Could you check a few things on this model? Use its own coordinates, in mm. A direction names the side the tool comes from. Coordinates: 2 decimals unless noted, no trailing zeros. Write each loop counter-clockwise with the first axis right and the second up, starting at its lowest first coordinate (ties: lowest second). Pieces come first, ordered by that corner, then holes.
```python
from build123d import *

# Parameters (mm, degrees)
SCHIZZO1_W                   = 12
SCHIZZO1_H                   = 21
SCHIZZO1_W_2                 = 21
SCHIZZO1_W_3                 = 15.1
SCHIZZO1_H_2                 = 15.1
ESTRUSIONE_ESTRUSIONE1_DEPTH = 15
SCHIZZO2_R                   = 1.5
TAGLIO_ESTRUSIONE1_DEPTH     = 15
SCHIZZO3_R                   = 1.5
TAGLIO_ESTRUSIONE2_DEPTH     = 15


with BuildPart() as part:
    # Schizzo1 → Estrusione-Estrusione1 (new body)
    # profile 1 of 2: a face of its own
    with BuildSketch(Plane(origin=(0, 0, 0), x_dir=(0, 0, -1), z_dir=(1, 0, 0))):
        with Locations((-16.5, 0)):
            Rectangle(SCHIZZO1_W, SCHIZZO1_H)
    # profile 2 of 2: a face of its own
    with BuildSketch(Plane(origin=(0, 0, 0), x_dir=(0, 0, -1), z_dir=(1, 0, 0))):
        Rectangle(SCHIZZO1_W_2, SCHIZZO1_H)
        Rectangle(SCHIZZO1_W_3, SCHIZZO1_H_2, mode=Mode.SUBTRACT)
    extrude(amount=ESTRUSIONE_ESTRUSIONE1_DEPTH)

    # Schizzo2 → Taglio-Estrusione1 (cut)
    with BuildSketch(Plane(origin=(0, 10.5, 0), x_dir=(1, 0, 0), z_dir=(0, 1, 0))):
        with Locations(Location((7.5, -15.5, 0), (0, 0, 270))):
            Circle(SCHIZZO2_R)
    extrude(amount=-TAGLIO_ESTRUSIONE1_DEPTH, mode=Mode.SUBTRACT)

    # Schizzo3 → Taglio-Estrusione2 (cut)
    with BuildSketch(Plane.XZ.offset(10.5)):
        with Locations(Location((7.5, 19.5, 0), (0, 0, 270))):
            Circle(SCHIZZO3_R)
    extrude(amount=-TAGLIO_ESTRUSIONE2_DEPTH, mode=Mode.SUBTRACT)


solid = part.part
```
1. If we mould it in two halves opening along Z, with no side actions, what happens to faces 6 (the face through (7, -10.5, 6)), 7 (the face through (6.6, -3.1, 20.7)), 8 (the face through (7, 0, -10.5))? For each: pulls with the +Z half, pulls with the -Z half, needs draft (parallel to the pull), parting line crosses it, or undercut.
Verdict:
face 6: needs draft
face 7: undercut
face 8: pulls with the -Z half
2. For pin 1 (2.5 mm diameter, centred on x = 7.5, z = 15.5, fed in from +Y); pin 2 (1.5 mm diameter, centred on x = 7.5, z = 19, fed in from -Y), each with a flat end and sliding along its axis, tell me the tip position at first contact or that it passes through.
Verdict:
pin 1: stops at y = -4.5
pin 2: stops at y = 4.5
3. Please list where these lines run through material, in increasing order: line 1 along Z through (x, y) = (5.5, -6.25); line 2 along Y through (x, z) = (0.5, -3); line 3 along X through (y, z) = (-2.75, 19.5).
Verdict:
line 1: z = -10.5 to -7.55, 7.55 to 22.5
line 2: y = -10.5 to -7.55, 7.55 to 10.5
line 3: x = 0 to 6, 9 to 15
4. I want a section at D-D on x = 3.5. Please give me the cut outline in (y, z).
Verdict:
outline: (-10.5, -10.5) - (10.5, -10.5) - (10.5, 22.5) - (-10.5, 22.5) - close; hole (-7.55, -7.55) - (7.55, -7.55) - (7.55, 7.55) - (-7.55, 7.55) - close
5. I want a section at B-B on z = 7. Please give me the cut outline in (x, y).
Verdict:
outline: (0, -10.5) - (15, -10.5) - (15, -7.55) - (0, -7.55) - close; (0, 7.55) - (15, 7.55) - (15, 10.5) - (0, 10.5) - close
6. I want a section at A-A on y = -5.25. Please give me the cut outline in (x, z), plus the area to 3 significant figures.
Verdict:
outline: (0, -10.5) - (15, -10.5) - (15, -7.55) - (0, -7.55) - close; (0, 7.55) - (15, 7.55) - (15, 22.5) - (0, 22.5) - close; hole circle Ø3 at (7.5, 19.5)
area: 261 mm2
7. On a 3-axis mill with a long thin cutter (end or side, diameter ignored), from which of +Z, -Z, +X, -X, +Y, -Y can I reach the whole of each face in a straight line? I mean faces 1 (the face through (8, 4.5, 20)), 2 (the face through (8, -4.5, 15)), 3 (the face through (0, 0, 10)), 4 (the face through (7, 0, 22.5)), 5 (the face through (7, 0, 7.55)). Say none if no direction works.
Verdict:
face 1: -Y
face 2: +Y
face 3: +Z, -Z, -X, +Y, -Y
face 4: +Z, +X, -X, +Y, -Y
face 5: +X, -X
8. I want a section at C-C on y = 2.5. Please give me the cut outline in (x, z), plus the area to 3 significant figures.
Verdict:
outline: (0, -10.5) - (15, -10.5) - (15, -7.55) - (0, -7.55) - close; (0, 7.55) - (15, 7.55) - (15, 22.5) - (0, 22.5) - close; hole circle Ø3 at (7.5, 15.5); hole circle Ø3 at (7.5, 19.5)
area: 254 mm2
